Could you check a few things on this model? Use its own coordinates, in mm. Face numbers are marked on the shaded views. A direction names the side the tool comes from. Coordinates: 2 decimals unless noted, no trailing zeros. Loops run counter-clockwise (first coordinate to the right, second up) from the corner with the lowest first, then second, coordinate; pieces in that order, holes last.
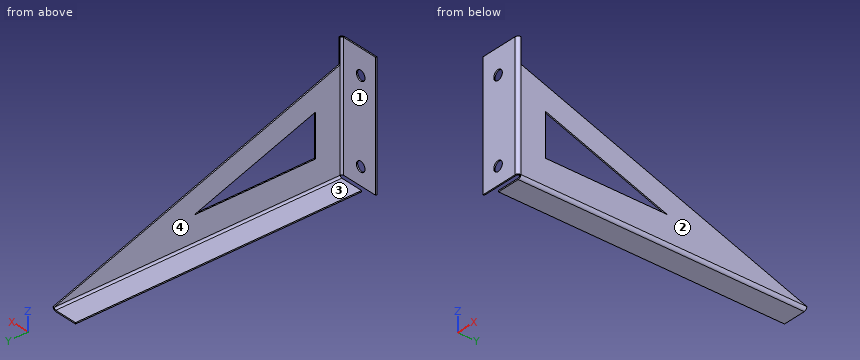
from build123d import *

# Parameters (mm, degrees)
SKETCH2_W          = 15
SKETCH2_H          = 50
BASE_FLANGE1_DEPTH = 0.5
EDGE_FLANGE1_DEPTH = 50
CUT_EXTRUDE1_DEPTH = 10
CUT_EXTRUDE2_DEPTH = 10
SKETCH22_R         = 2
CUT_EXTRUDE3_DEPTH = 10
EDGE_FLANGE2_DEPTH = 115.2634


# Sheet-metal steps are written as plain solids
with BuildPart() as part:
    # Sketch2 → Base-Flange1 (new body)
    with BuildSketch(Plane(origin=(0, 0, 0), x_dir=(1, 0, 0), z_dir=(0, 1, 0))):
        with Locations((-7.5, -25)):
            Rectangle(SKETCH2_W, SKETCH2_H)
    extrude(amount=-BASE_FLANGE1_DEPTH)

    # Edge-Flange1 section (across the edge) → Edge-Flange1 (add)
    with BuildSketch(Plane(origin=(0.7366, 0, 50), x_dir=(-1, 0, 0), z_dir=(0, 0, -1))):
        with BuildLine():
            Line((-0.5, 0.7366), (-0.5, 116))
            Line((-0.5, 116), (0, 116))
            Line((0, 116), (0, 0.7366))
            ThreePointArc((0, 0.7366), (0.215745145, 0.215745145), (0.7366, 0))
            Line((0.7366, 0), (0.7366, -0.5))
            ThreePointArc((0.7366, -0.5), (-0.137808246, -0.137808246), (-0.5, 0.7366))
        make_face()
    extrude(amount=EDGE_FLANGE1_DEPTH)

    # Sketch19 → Cut-Extrude1 (cut)
    with BuildSketch(Plane.ZY.offset(-0.7366)):
        Polygon((50, 0.7366), (40, 0.7366), (0, 116), (50, 116), align=None)
    extrude(amount=-CUT_EXTRUDE1_DEPTH, mode=Mode.SUBTRACT)

    # Sketch21 → Cut-Extrude2 (cut)
    with BuildSketch(Plane.ZY.offset(-0.7366)):
        Polygon((10, 10.7366), (10, 59.7366), (27, 10.7366), align=None)
    extrude(amount=-CUT_EXTRUDE2_DEPTH, mode=Mode.SUBTRACT)

    # Sketch22 → Cut-Extrude3 (cut)
    with BuildSketch(Plane(origin=(0, 0, 0), x_dir=(1, 0, 0), z_dir=(0, 1, 0))):
        with Locations(Location((-8, -40, 0), (0, 0, 270))):
            Circle(SKETCH22_R)
        with Locations(Location((-8, -7, 0), (0, 0, 270))):
            Circle(SKETCH22_R)
    extrude(amount=-CUT_EXTRUDE3_DEPTH, mode=Mode.SUBTRACT)

    # Edge-Flange2 section (across the edge) → Edge-Flange2 (add)
    with BuildSketch(Plane(origin=(0.7366, 116, -0.7366), x_dir=(0, 0, 1), z_dir=(0, -1, 0))):
        with BuildLine():
            Line((-0.5, 0.7366), (-0.5, 10))
            Line((-0.5, 10), (0, 10))
            Line((0, 10), (0, 0.7366))
            ThreePointArc((0, 0.7366), (0.215745145, 0.215745145), (0.7366, 0))
            Line((0.7366, 0), (0.7366, -0.5))
            ThreePointArc((0.7366, -0.5), (-0.137808246, -0.137808246), (-0.5, 0.7366))
        make_face()
    extrude(amount=EDGE_FLANGE2_DEPTH)


solid = part.part
(1) Imagine slicing it at B-B, the plane x = -8. Write out the boundary of the cut face in (y, z), and give its area (3 significant figures).
Answers:
outline: (-0.5, 0) - (0, 0) - (0, 5) - (-0.5, 5) - close; (-0.5, 9) - (0, 9) - (0, 38) - (-0.5, 38) - close; (-0.5, 42) - (0, 42) - (0, 50) - (-0.5, 50) - close; (0.74, -1.24) - (116, -1.24) - (116, -0.74) - (0.74, -0.74) - close
area: 78.6 mm2
(2) Imagine slicing it at C-C, the plane z = 46. Write out the boundary of the cut face in (x, y), and give its area (3 significant figures).
Answers:
outline: (-15, -0.5) - (0, -0.5) arc R1.24 ccw to (1.24, 0.74) - (0.74, 0.74) arc R0.74 cw to (0, 0) - (-15, 0) - close
area: 8.27 mm2
(3) Imagine slicing it at A-A, the plane x = -3. Write out the boundary of the cut face in (y, z).
Answers:
outline: (-0.5, 0) - (0, 0) - (0, 50) - (-0.5, 50) - close; (0.74, -1.24) - (116, -1.24) - (116, -0.74) - (0.74, -0.74) - close
(4) I need wall thicknesses on probe 1 along Y at (x, z) = (-6, 24.5); probe 2 along Z at (x, y) = (-9, 92.5); probe 3 along X at (y, z) = (42.5, 23.5). Which ranges of each line are inside material? Lowest first, please.
Answers:
probe 1: y = -0.5 to 0
probe 2: z = -1.24 to -0.74
probe 3: x = 0.74 to 1.24
(5) Which directions (+Z, -Z, +X, -X, +Y, -Y) give clear straight access to the entire face, cutting with the end or side of a thin tool? Please do the marked faces 1, 2, 3 and 4.
Answers:
face 1: +Z, -Z, -X, +Y
face 2: +Z, -Z, +X, +Y, -Y
face 3: +Z, -X, +Y, -Y
face 4: +Z, -X, +Y
(6) Imagine slicing it at D-D, the plane y = 54.5. Write out the boundary of the cut face in (x, z), and give its area (3 significant figures).
Answers:
outline: (-9.26, -1.24) - (0, -1.24) arc R1.24 ccw to (1.24, 0) - (1.24, 10) - (0.74, 10) - (0.74, 0) arc R0.74 cw to (0, -0.74) - (-9.26, -0.74) - close; (0.74, 11.82) - (1.24, 11.82) - (1.24, 21.34) - (0.74, 21.34) - close
area: 15.2 mm2
(7) For pin 1 (1 mm diameter, centred on x = -4, y = 0, fed in from -Z); pin 2 (2.5 mm diameter, centred on x = -8, z = 40, fed in from -Y); pin 3 (7.5 mm diameter, centred on x = -2.5, y = 40, fed in from +Z); pin 4 (4.5 mm diameter, centred on x = -7.5, z = 26, fed in from +Y), each with a flat end and sliding along its axis, tell me the tip position at first contact or that it passes through.
Answers:
pin 1: stops at z = 0
pin 2: passes through
pin 3: stops at z = 27.03
pin 4: stops at y = 0
